Here's how the part is built. I have some questions about the finished solid (model axes, mm). Face numbers are marked on the shaded views. Coordinates: 2 decimals unless noted, no trailing zeros. Loops run counter-clockwise (first coordinate to the right, second up) from the corner with the lowest first, then second, coordinate; pieces in that order, holes last. Notation, with made-up numbers: (65.25, 13.25) -> (86.25, 13.25) arc R26 ccw to (86.25, 47.25) -> close; hole circle Ø11 at (72.5, 67). An arc over 180 degrees is marked (long way). Answer as a JSON object with one key per item and string values. Group by question number.
Q1. I want a section at B-B on y = 1.25. Write out the boundary of the cut face in (x, z), then the cut area to 3 significant figures.
Q2. I'm going to push flat-ended pins straight in: pin 1 (6 mm diameter, centred on x = 1, z = 1, fed in from +Y); pin 2 (3 mm diameter, centred on x = 1, z = -3.5, fed in from -Y); pin 3 (0.5 mm diameter, centred on x = 3.5, y = 0.5, fed in from +Z); pin 4 (5 mm diameter, centred on x = 2.5, z = 2.5, fed in from +Y). Where does each tip first touch, or does it pass through?
Q3. I want a section at A-A on z = -4. Write out the boundary of the cut face in (x, y).
Q4. I want a section at D-D on y = 0.2. Write out the boundary of the cut face in (x, z).
Q5. I want a section at C-C on x = 1.5. Write out the boundary of the cut face in (y, z), then the cut area to 3 significant figures.
Q6. Thinking about a two-plate mould opening in X: for the marked faces 1, 2 and 3, which applies, released by +X, released by -X, zero draft, split by the parting line, or undercut?
Q7. I need wall thicknesses on line 1 (Z direction, x = -3, y = 0.15); line 2 (Y direction, x = 2.75, z = -3); line 3 (Y direction, x = 2.25, z = -4.5). Which ranges of each line are inside material? Lowest first, please.
```python
from build123d import *

# Parameters (mm, degrees)
BASE_DEPTH         = 0.5
BACK_HEIGHT_DEPTH  = 1
FRONT_HEIGHT_DEPTH = 0.5


with BuildPart() as part:
    # Sketch1 → Base (new body)
    with BuildSketch(Plane(origin=(0, 0, 0), x_dir=(1, 0, 0), z_dir=(0, 1, 0))):
        with BuildLine():
            Line((2.3, 5.15), (5.15, 2.3))
            Line((5.15, 2.3), (5.15, 0.6))
            Line((5.15, 0.6), (1.75, 0.6))
            ThreePointArc((1.75, 0.6), (1.15, 0), (1.75, -0.6))
            Line((1.75, -0.6), (5.15, -0.6))
            Line((5.15, -0.6), (5.15, -2.3))
            Line((5.15, -2.3), (2.3, -5.15))
            Line((2.3, -5.15), (-5.15, -5.15))
            Line((-5.15, -5.15), (-5.15, -0.6))
            Line((-5.15, -0.6), (-1.75, -0.6))
            ThreePointArc((-1.75, -0.6), (-1.15, 0), (-1.75, 0.6))
            Line((-1.75, 0.6), (-5.15, 0.6))
            Line((-5.15, 0.6), (-5.15, 5.15))
            Line((-5.15, 5.15), (2.3, 5.15))
        make_face()
    extrude(amount=BASE_DEPTH)

    # Sketch2 → Back Height (add)
    with BuildSketch(Plane(origin=(0, 0.5, 0), x_dir=(1, 0, 0), z_dir=(0, 1, 0))):
        with BuildLine():
            Line((-0.6, 4.963869458), (-0.6, 5.15))
            Line((-0.6, 5.15), (-5.15, 5.15))
            Line((-5.15, 5.15), (-5.15, 0.6))
            Line((-5.15, 0.6), (-4.963869458, 0.6))
            ThreePointArc((-4.963869458, 0.6), (-3.535533906, 3.535533906), (-0.6, 4.963869458))
        make_face()
        with BuildLine():
            ThreePointArc((-0.6, -4.963869458), (-3.535533906, -3.535533906), (-4.963869458, -0.6))
            Line((-4.963869458, -0.6), (-5.15, -0.6))
            Line((-5.15, -0.6), (-5.15, -5.15))
            Line((-5.15, -5.15), (-0.6, -5.15))
            Line((-0.6, -5.15), (-0.6, -4.963869458))
        make_face()
    extrude(amount=BACK_HEIGHT_DEPTH)

    # Sketch2<3> → Front Height (add)
    with BuildSketch(Plane(origin=(0, 0.5, 0), x_dir=(1, 0, 0), z_dir=(0, 1, 0))):
        with BuildLine():
            Line((2.3, 5.15), (0.6, 5.15))
            Line((0.6, 5.15), (0.6, 4.963869458))
            ThreePointArc((0.6, 4.963869458), (3.535533906, 3.535533906), (4.963869458, 0.6))
            Line((4.963869458, 0.6), (5.15, 0.6))
            Line((5.15, 0.6), (5.15, 2.3))
            Line((5.15, 2.3), (2.3, 5.15))
        make_face()
        with BuildLine():
            Line((5.15, -0.6), (4.963869458, -0.6))
            ThreePointArc((4.963869458, -0.6), (3.535533906, -3.535533906), (0.6, -4.963869458))
            Line((0.6, -4.963869458), (0.6, -5.15))
            Line((0.6, -5.15), (2.3, -5.15))
            Line((2.3, -5.15), (5.15, -2.3))
            Line((5.15, -2.3), (5.15, -0.6))
        make_face()
    extrude(amount=FRONT_HEIGHT_DEPTH)


solid = part.part
```
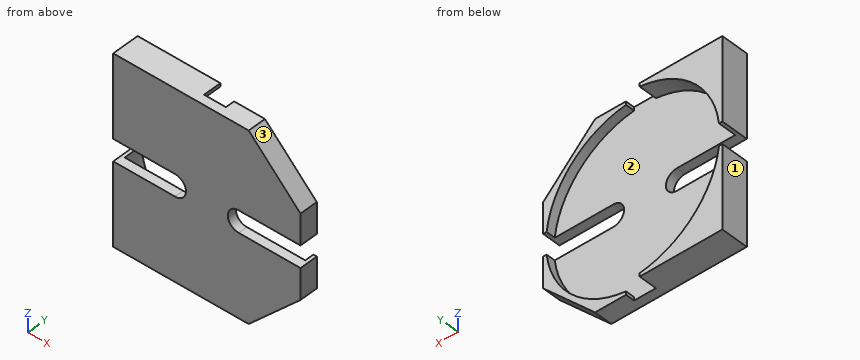
Result set:
{
 "1": {"outline": "(-5.15, -5.15) -> (-0.6, -5.15) -> (-0.6, -4.96) arc R5 cw to (-4.96, -0.6) -> (-5.15, -0.6) -> close; (-5.15, 0.6) -> (-4.96, 0.6) arc R5 cw to (-0.6, 4.96) -> (-0.6, 5.15) -> (-5.15, 5.15) -> close", "area": "13.4 mm²"},
 "2": {"pin 1": "stops at y = 0.5", "pin 2": "stops at y = 0", "pin 3": "stops at z = 4.2", "pin 4": "stops at y = 1"},
 "3": {"outline": "(-5.15, 0) -> (3.45, 0) -> (3.45, 1) -> (3, 1) -> (3, 0.5) -> (-3, 0.5) -> (-3, 1.5) -> (-5.15, 1.5) -> close"},
 "4": {"outline": "(-5.15, -5.15) -> (2.3, -5.15) -> (5.15, -2.3) -> (5.15, -0.6) -> (1.75, -0.6) arc R0.6 cw to (1.75, 0.6) -> (5.15, 0.6) -> (5.15, 2.3) -> (2.3, 5.15) -> (-5.15, 5.15) -> (-5.15, 0.6) -> (-1.75, 0.6) arc R0.6 cw to (-1.75, -0.6) -> (-5.15, -0.6) -> close"},
 "5": {"outline": "(0, -5.15) -> (1, -5.15) -> (1, -4.77) -> (0.5, -4.77) -> (0.5, -0.55) -> (0, -0.55) -> close; (0, 0.55) -> (0.5, 0.55) -> (0.5, 4.77) -> (1, 4.77) -> (1, 5.15) -> (0, 5.15) -> close", "area": "4.98 mm²"},
 "6": {"face 1": "released by -X", "face 2": "undercut", "face 3": "released by +X"},
 "7": {"line 1": "z = -5.15 to -0.6, 0.6 to 5.15", "line 2": "y = 0 to 0.5", "line 3": "y = 0 to 1"}
}
